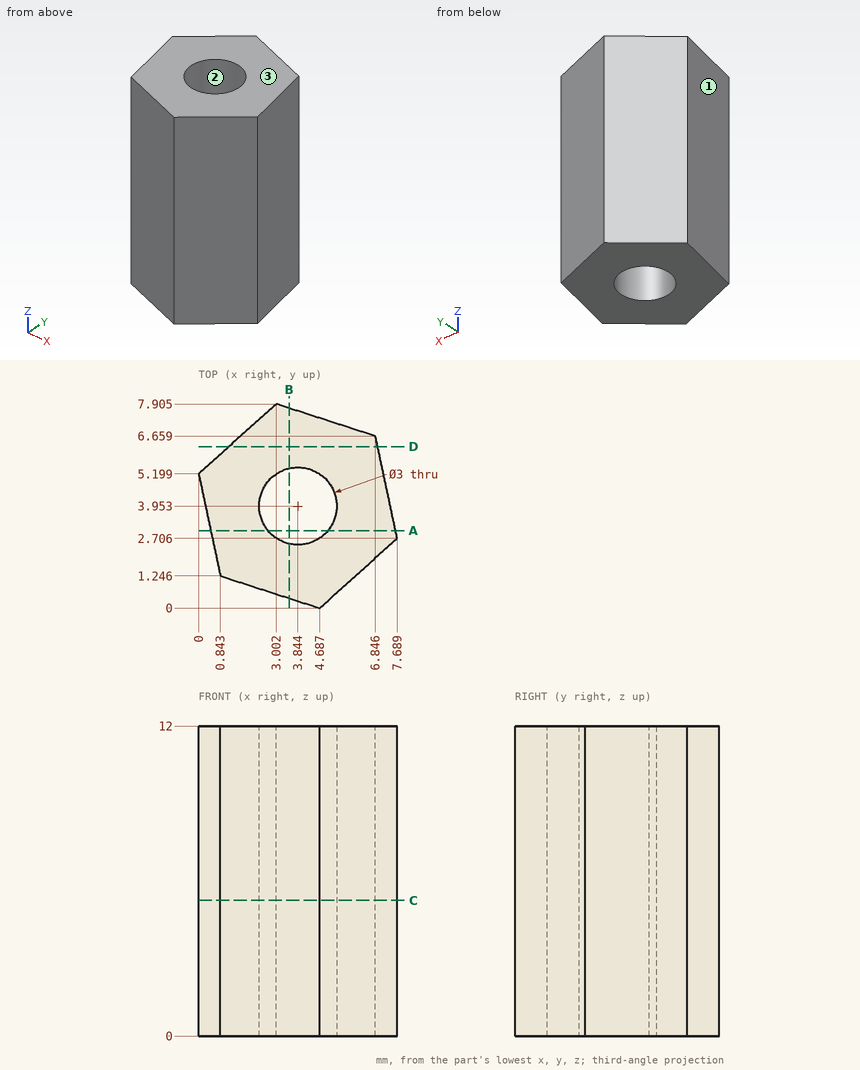
Study the drawing (mm; zero at the part's minimum x, y, z) and answer. Round coordinates to 2 decimals unless told otherwise and drop trailing zeros. Loops run counter-clockwise (first coordinate to the right, second up) from the corner with the lowest first, then second, coordinate; pieces in that order, holes last. Notation, with made-up numbers: (70, 73.5) -> (95, 73.5) arc R14 ccw to (95, 91.5) -> close; hole circle Ø9 at (-5, 51). An arc over 180 degrees is marked (long way). Use one line per item in the form item = value.
1. The part is cut by section D-D on y = 6.25. Determine the outline of the cut face in (x, z) (1 decimal), and give its area (3 significant figures).
Answer key:
outline = (1.2, 0) -> (6.9, 0) -> (6.9, 12) -> (1.2, 12) -> close
area = 69.2 mm²
2. Find the intervals of material crossed by probe 1 along Y at (x, z) = (5, 10.5) (1 decimal); probe 2 along Y at (x, z) = (3.25, 6.75) (1 decimal); probe 3 along X at (y, z) = (3, 10) (1 decimal), in increasing order. Write a range as [from, to].
Answer key:
probe_1 = [0.3, 3], [4.9, 7.3]
probe_2 = [0.5, 2.6], [5.3, 7.8]
probe_3 = [0.5, 2.7], [5, 7.6]
3. For a pull along X with two mould halves and no side action, classify the marked faces 1, 2 and 3 as released by +X, released by -X, zero draft, split by the parting line, or undercut.
Answer key:
face_1 = released by -X
face_2 = undercut
face_3 = zero draft
4. The part is cut by section C-C on z = 5.25. Determine the outline of the cut face in (x, y) (1 decimal).
Answer key:
outline = (0, 5.2) -> (0.8, 1.2) -> (4.7, 0) -> (7.7, 2.7) -> (6.8, 6.7) -> (3, 7.9) -> close; hole circle Ø3 at (3.8, 4)
5. Flat-ended cylindrical pins translate along their axes: pin 1 Ø1.5 at (x, z) = (5, 3) entering from +Y; pin 2 Ø1 at (x, z) = (4, 6.5) entering from +Y; pin 3 Ø3 at (y, z) = (3.5, 7.5) entering from -X. Find the tip coordinate at first contact, or state that the pin passes through.
Answer key:
pin_1 = 7.5
pin_2 = 7.74
pin_3 = 0.04
6. The part is cut by section B-B on x = 3.5. Determine the outline of the cut face in (y, z) (1 decimal).
Answer key:
outline = (0.4, 0) -> (2.5, 0) -> (2.5, 12) -> (0.4, 12) -> close; (5.4, 0) -> (7.7, 0) -> (7.7, 12) -> (5.4, 12) -> close
7. The part is cut by section A-A on y = 3. Determine the outline of the cut face in (x, z) (1 decimal).
Answer key:
outline = (0.5, 0) -> (2.7, 0) -> (2.7, 12) -> (0.5, 12) -> close; (5, 0) -> (7.6, 0) -> (7.6, 12) -> (5, 12) -> close
